Input: part model. Units: mm. Frame: model coordinates. Face numbers are marked on the shaded views. A direction names the side the tool comes from. Give positions to 0.01 mm unless a question says otherwise; leave off trailing zeros. Write each loop counter-clockwise with the first axis right and the second up, starting at its lowest first coordinate (ties: lowest second). Pieces come first, ordered by that corner, then holes. Notation, with made-up numbers: (68, 24) - (79, 24) arc R20 cw to (79, 55) - close; hole circle Ø4 at (-29, 18). An arc over 180 degrees is marked (long way). Use a Markdown table: item, result. Add a question column.
1. Material intervals for probe 1 along Y at (x, z) = (7.75, -0.75); probe 2 along Z at (x, y) = (7.75, 2.25); probe 3 along Z at (x, y) = (-7.25, -4.5), sorted ascending.
2. Section query D-D, the plane y = -8. Return loops of the section in (x, z).
3. Pin query (flat end, axial travel): pin 1 (1.5 mm diameter, centred on x = -2.5, z = 3, fed in from +Y); pin 2 (2.5 mm diameter, centred on x = 10, z = -2, fed in from -Y); pin 3 (8 mm diameter, centred on x = 4.5, y = -8, fed in from -Z); pin 4 (0.9 mm diameter, centred on y = 3.5, z = -1.5, fed in from -X). Return the tip coordinate at first contact, or that it passes through.
4. Set-up query: the marked faces 1, 2, 3 and 4. Return all of +Z, -Z, +X, -X, +Y, -Y with unobstructed straight access to the full face (end or side cutting, diameter ignored); none if empty.
5. Section query C-C, the plane z = -1.25. Return loops of the section in (x, y).
6. Section query A-A, the plane x = -5. Return loops of the section in (y, z).
7. Section query B-B, the plane y = -2.75. Return loops of the section in (x, z), plus the area to 3 significant figures.
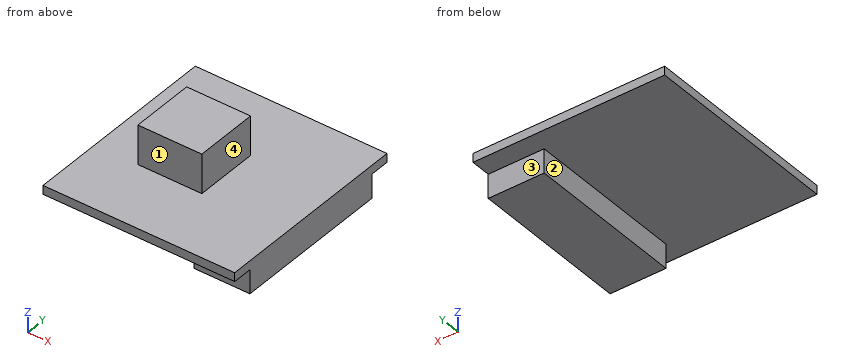
```python
from build123d import *

# Parameters (mm, degrees)
F0_W     = 8
F0_H     = 8
F0_W_2   = 7
F0_H_2   = 20
F1_DEPTH = 1.1
F2_DEPTH = 6
F3_DEPTH = 3


with BuildPart() as f1:
    # F0 (on Top) → F1 (new body)
    with BuildSketch(Plane.XY):
        Polygon((12, 12.5), (-12, 12.5), (-12, -12.5), (12, -12.5), (12, -10), (5, -10), (5, 10), (12, 10), align=None)
        with Locations((-2.6, 0)):
            Rectangle(F0_W, F0_H, mode=Mode.SUBTRACT)
        with Locations((-2.6, 0)):
            Rectangle(F0_W, F0_H)
        with Locations((8.5, 0)):
            Rectangle(F0_W_2, F0_H_2)
    extrude(amount=F1_DEPTH)

    # F0 (on Top) → F2 (join)
    with BuildSketch(Plane.XY):
        with Locations((-2.6, 0)):
            Rectangle(F0_W, F0_H)
    extrude(amount=F2_DEPTH)

    # F0 (on Top) → F3 (join)
    with BuildSketch(Plane.XY):
        with Locations((8.5, 0)):
            Rectangle(F0_W_2, F0_H_2)
    extrude(amount=-F3_DEPTH)


solid = f1.part
```
Result sheet:
| question | item | result |
|---|---|---|
| 1 | probe 1 | y = -10 to 10 |
| 1 | probe 2 | z = -3 to 1.1 |
| 1 | probe 3 | z = 0 to 1.1 |
| 2 | outline | (-12, 0) - (5, 0) - (5, -3) - (12, -3) - (12, 1.1) - (-12, 1.1) - close |
| 3 | pin 1 | stops at y = 4 |
| 3 | pin 2 | stops at y = -10 |
| 3 | pin 3 | stops at z = -3 |
| 3 | pin 4 | stops at x = 5 |
| 4 | face 1 | +Z, +X, -X, -Y |
| 4 | face 2 | -Z, -X, +Y, -Y |
| 4 | face 3 | -Z, +X, -X, +Y |
| 4 | face 4 | +Z, +X, +Y, -Y |
| 5 | outline | (5, -10) - (12, -10) - (12, 10) - (5, 10) - close |
| 6 | outline | (-12.5, 0) - (12.5, 0) - (12.5, 1.1) - (4, 1.1) - (4, 6) - (-4, 6) - (-4, 1.1) - (-12.5, 1.1) - close |
| 7 | outline | (-12, 0) - (5, 0) - (5, -3) - (12, -3) - (12, 1.1) - (1.4, 1.1) - (1.4, 6) - (-6.6, 6) - (-6.6, 1.1) - (-12, 1.1) - close |
| 7 | area | 86.6 mm² |
